```python
from build123d import *

# Parameters (mm, degrees)
F0_W     = 50.8
F0_H     = 25.4
F0_W_2   = 44.45
F0_H_2   = 19.05
F1_DEPTH = 101.6
F3_D     = 5.1054
F5_D     = 5.1054


# Not quite as in the source:
# - a feature names something its author has since deleted; it is built from what else it names


with BuildPart() as f1:
    # F0 (on Front) → F1 (new body)
    with BuildSketch(Plane.XZ):
        Rectangle(F0_W, F0_H)
        Rectangle(F0_W_2, F0_H_2, mode=Mode.SUBTRACT)
    extrude(amount=F1_DEPTH)

    # F3 (through all)
    with Locations(Plane.XY.offset(12.7)):
        with Locations((-12.7, -88.9), (-12.7, -12.7), (-12.7, -38.1), (-12.7, -63.5), (12.7, -12.7), (12.7, -88.9), (12.7, -38.1), (12.7, -63.5)):
            Hole(F3_D / 2)

    # F5 (through all)
    with Locations(Plane.YZ.offset(25.4)):
        with Locations((-88.9, 0), (-63.5, 0), (-38.1, 0), (-12.7, 0)):
            Hole(F5_D / 2)


solid = f1.part
```
Build history of the part. All positions in model axes, mm. A direction names the side the tool comes from. Round coordinates to 2 decimals unless told otherwise and drop trailing zeros. Loops run counter-clockwise (first coordinate to the right, second up) from the corner with the lowest first, then second, coordinate; pieces in that order, holes last.
Item 1: Drill centre lines: line 1 along Y through (x, z) = (12.7, -10.25); line 2 along X through (y, z) = (-52.5, 1.5) (3 decimals); line 3 along Z through (x, y) = (10, -36.5) (3 decimals). Where is each one in solid material? Low to high.
Item 2: Which spindle directions (+Z, -Z, +X, -X, +Y, -Y) get a long thin tool onto all of the face, cutting with end or side? Do faces 4 (the face through (-22.225, -50, 0)), 5 (the face through (-23.835, -15.135, 0.767)). Say none if no direction does.
Item 3: Saw through at B-B (y = -77). List the corners of the cut face in (x, z) (3 decimals).
Item 4: Two-plate mould, pull along Y, no slides. Class faces 1 (the face through (0, -101.6, 10)), 2 (the face through (0, 0, 10)), 3 (the face through (-13.878, -65.765, 11.09)): released by +Y, released by -Y, zero draft, split by the parting line, or undercut.
Item 5: Saw through at C-C (y = -88.9). State how many separate pieces and enclosed holes the cut face has, then the cut area to 3 significant figures.
Item 6: Saw through at A-A (x = 8). List the corners of the cut face in (y, z) (3 decimals), then the cut area to 3 significant figures.
Item 7: Pin check, flat tip, straight feed: P1, Ø8, axis at y = -88.9, z = 0, coming from the +X side. Stop position of the tip, or through.
Item 8: Saw through at D-D (z = -4.5). List the corners of the cut face in (x, y) (3 decimals), then the cut area to 3 significant figures.
Worked answers:
1. line 1: y = -101.6 to -91.45, -86.35 to -66.05, -60.95 to -40.65, -35.55 to -15.25, -10.15 to 0
1. line 2: x = -25.4 to -22.225, 22.225 to 25.4
1. line 3: z = -12.7 to -9.525, 9.525 to 12.7
2. face 4: +Y, -Y
2. face 5: +X, -X
3. outline: (-25.4, -12.7) - (25.4, -12.7) - (25.4, 12.7) - (-25.4, 12.7) - close; hole (-22.225, -9.525) - (22.225, -9.525) - (22.225, 9.525) - (-22.225, 9.525) - close
4. face 1: released by -Y
4. face 2: released by +Y
4. face 3: undercut
5. separate pieces: 6
5. enclosed holes: 0
5. area: 346 mm2
6. outline: (-101.6, -12.7) - (0, -12.7) - (0, -9.525) - (-101.6, -9.525) - close; (-101.6, 9.525) - (0, 9.525) - (0, 12.7) - (-101.6, 12.7) - close
6. area: 645 mm2
7. P1: stops at x = 25.4
8. outline: (-25.4, -101.6) - (-22.225, -101.6) - (-22.225, 0) - (-25.4, 0) - close; (22.225, -101.6) - (25.4, -101.6) - (25.4, 0) - (22.225, 0) - close
8. area: 645 mm2
